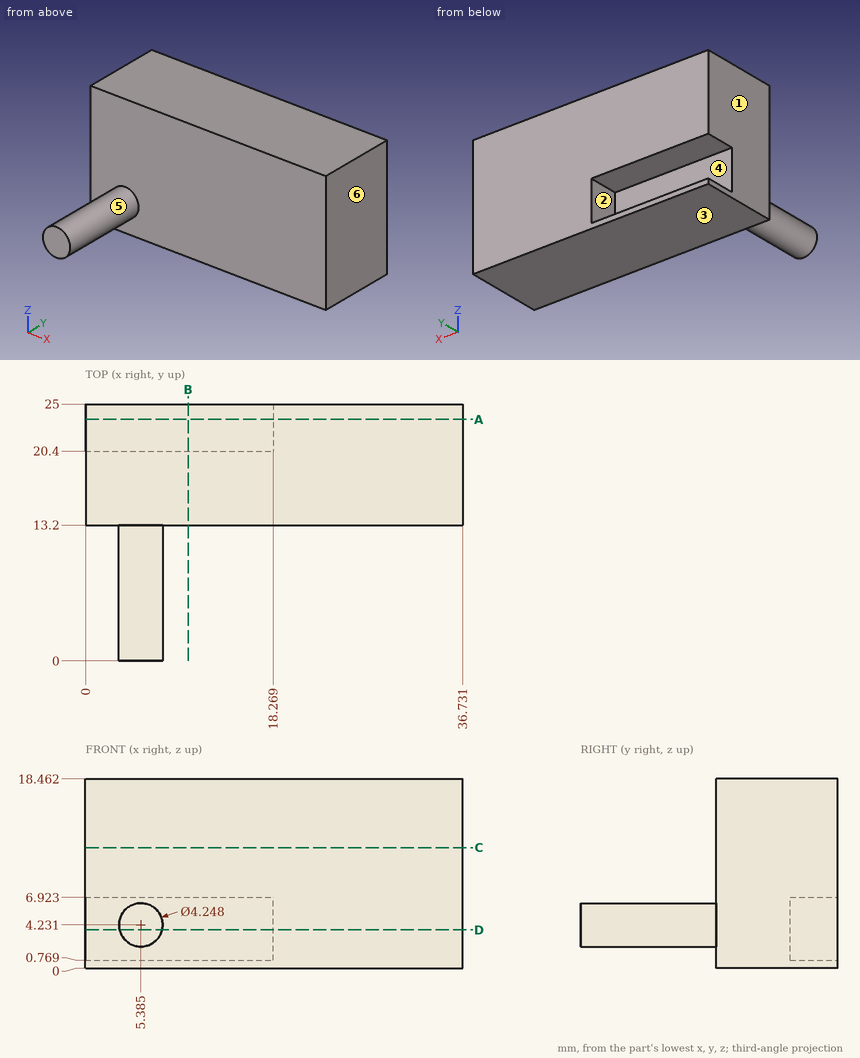
Geometry check sheet. Reference: drawing and pictorial views, mm from the part's lowest x, y, z. A direction names the side the tool comes from. Give positions to 0.01 mm unless a question says otherwise; leave off trailing zeros. Order: outer loops, then holes, each group sorted by start corner. A loop starts at its lowest first (then second) coordinate and runs counter-clockwise, first axis right, second up. Notation, with made-up numbers: M -32.5,67 L -4.5,67 A10 ccw -4.5,72 Z; hole C 48.25,-22 d4. An arc over 180 degrees is marked long. Answer as a JSON object with one key per item and string values. Group by question number.
1) Cross-section at B-B (x = 10). Enter the section's corners in (y, z).
2) Depth check by flat-ended pin: pin 1 Ø2.5 at (y, z) = (23.5, 2.5) entering from -X; pin 2 Ø9 at (x, z) = (15, 10) entering from -Y. Enter the tip coordinate at first touch or a pass-through.
3) Scan lines: line 1 along Z through (x, y) = (3, 22.5); line 2 along Y through (x, z) = (28, 2.75). Record each from-to range of solid material in increasing order. Write a range as [from, to].
4) Access from +Z, -Z, +X, -X, +Y, -Y to the whole of each face (thin tool, end or side, straight path). Record for the marked faces 4, 5 and 6.
5) Cross-section at D-D (z = 3.75). Enter the section's corners in (x, y) (1 decimal).
6) Cross-section at C-C (z = 11.75). Enter the section's corners in (x, y).
7) Mould release check, pull along Z, two halves, no side actions. Record for the marked faces 1, 2 and 3: released by +Z, released by -Z, zero draft, split by the parting line, or undercut.
8) Cross-section at A-A (y = 23.5). Enter the section's corners in (x, z).
Result sheet:
{
 "1": {"outline": "M 13.2,0 L 25,0 L 25,0.77 L 20.4,0.77 L 20.4,6.92 L 25,6.92 L 25,18.46 L 13.2,18.46 Z"},
 "2": {"pin 1": "stops at x = 18.27", "pin 2": "stops at y = 13.2"},
 "3": {"line 1": "z = [0, 0.77], [6.92, 18.46]", "line 2": "y = [13.2, 25]"},
 "4": {"face 4": "-X, +Y", "face 5": "-Y", "face 6": "+Z, -Z, +X, +Y, -Y"},
 "5": {"outline": "M 0,13.2 L 3.3,13.2 L 3.3,0 L 7.5,0 L 7.5,13.2 L 36.7,13.2 L 36.7,25 L 18.3,25 L 18.3,20.4 L 0,20.4 Z"},
 "6": {"outline": "M 0,13.2 L 36.73,13.2 L 36.73,25 L 0,25 Z"},
 "7": {"face 1": "zero draft", "face 2": "undercut", "face 3": "released by -Z"},
 "8": {"outline": "M 0,0 L 36.73,0 L 36.73,18.46 L 0,18.46 L 0,6.92 L 18.27,6.92 L 18.27,0.77 L 0,0.77 Z"}
}
